Part print with two shaded views. Sizes in mm from the minimum x, y, z corner. A direction names the side the tool comes from. Coordinates: 2 decimals unless noted, no trailing zeros. Loops run counter-clockwise (first coordinate to the right, second up) from the corner with the lowest first, then second, coordinate; pieces in that order, holes last.
(1) Two-plate mould, pull along X, no slides. Class the marked faces 4, 5 and 6: pulls with the +X half, pulls with the -X half, needs draft (parallel to the pull), parting line crosses it, or undercut.
(2) Wall check: L1, parallel to Y at x = 38.5, z = 71; L2, parallel to Z at x = 22, y = 556; L3, parallel to Y at x = 69, z = 32. Give the ranges that are in metal, low to high.
(3) Tool access for the marked faces 1, 2 and 3: list every direction of +Z, -Z, +X, -X, +Y, -Y with a clear straight run to the whole face (end or side of a thin tool).
(4) Slice it at A-A (x = 29). Give the cut face in (y, z).
(5) Slice it at B-B (z = 68.5). Give the cut face in (x, y).
(6) Flat gauge pins, fed straight in: P1, Ø22, axis at x = 50, z = 66.5, coming from the +Y side; P2, Ø5, axis at x = 57.5, z = 14, coming from the -Y side; P3, Ø4, axis at x = 35, z = 22, coming from the -Y side. Where does each tip first touch, or does it go through?
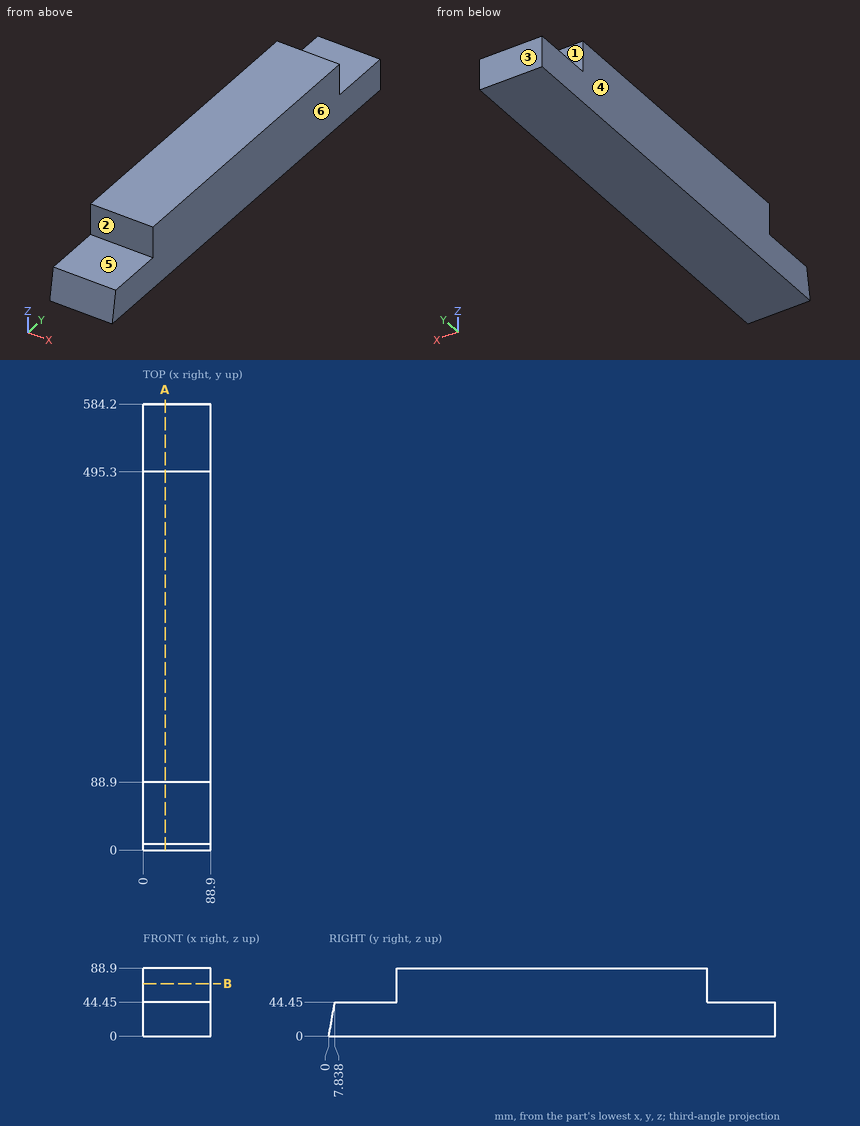
Response values:
1. face 4: pulls with the -X half
1. face 5: needs draft
1. face 6: pulls with the +X half
2. L1: y = 88.9 to 495.3
2. L2: z = 0 to 44.45
2. L3: y = 5.64 to 584.2
3. face 1: +Z, +X, -X, +Y
3. face 2: +Z, +X, -X, -Y
3. face 3: +Z, -Z, +X, -X, +Y
4. outline: (0, 0) - (584.2, 0) - (584.2, 44.45) - (495.3, 44.45) - (495.3, 88.9) - (88.9, 88.9) - (88.9, 44.45) - (7.84, 44.45) - close
5. outline: (0, 88.9) - (88.9, 88.9) - (88.9, 495.3) - (0, 495.3) - close
6. P1: stops at y = 495.3
6. P2: stops at y = 2.03
6. P3: stops at y = 3.53
